Autodesk Inventor part; units mm, degrees
ref_plane "C3_XY" through (128, 0, 0) normal (-1, 0, 0) x (0, 0, -1)
ref_plane "C3_YZ" through (128, 0, 0) normal (0, 0, -1) x (0, -1, 0)
ref_plane "C3_ZX" through (128, 0, 0) normal (0, -1, 0) x (-1, 0, 0)
sketch "Sketch_1" plane through (0, 0, 0) normal (0, 0, 1) x (1, 0, 0)
  line L0 (128, 0) -> (0, 0)
  line L1 (0, 0) -> (0, 3.5)
  line L2 (0, 3.5) -> (0.6062, 4.55)
  line L3 (0.6062, 4.55) -> (127.3938, 4.55)
  line L4 (127.3938, 4.55) -> (128, 3.5)
  line L5 (128, 3.5) -> (128, 0)
  line L6 (128, 0) -> (0, 0)
revolve "Revolution1" add sketch "Sketch_1" angle 360 about axis through (128, 0, 0) along (1, 0, 0)
sketch "Sketch_2" plane through (0, 0, 0) normal (1, 0, 0) x (0, 1, 0)
  line L0 (7, 7) -> (-7, 7)
  line L1 (-7, 7) -> (-7, -7)
  line L2 (-7, -7) -> (7, -7)
  line L3 (7, -7) -> (7, 7)
  line L4 (-2.0207, 3.5) -> (-4.0415, 0)
  line L5 (-4.0415, 0) -> (-2.0207, -3.5)
  line L6 (-2.0207, -3.5) -> (2.0207, -3.5)
  line L7 (2.0207, -3.5) -> (4.0415, 0)
  line L8 (4.0415, 0) -> (2.0207, 3.5)
  line L9 (2.0207, 3.5) -> (-2.0207, 3.5)
extrude "Extrusion1" cut sketch "Sketch_2" along normal blind 128
sketch "Sketch3" plane through (0, 0, 0) normal (-1, 0, 0) x (0, 0, 1)
  point P0 (0, 0)
hole "Hole1" at (0, 0, 0) direction (1, 0, 0) diameter 2.459 depth 8.2901 tip angle 120 countersink diameter 3 countersink angle 90
sketch "Sketch4" plane through (128, 0, 0) normal (1, 0, 0) x (0, 0, -1)
  point P0 (0, 0)
hole "Hole2" at (128, 0, 0) direction (-1, 0, 0) diameter 2.459 depth 8.2901 tip angle 120 countersink diameter 3 countersink angle 90
ref_plane "C3_XY" through (128, 0, 0) normal (-1, 0, 0) x (0, 0, -1)
ref_plane "C3_YZ" through (128, 0, 0) normal (0, 0, -1) x (0, -1, 0)
ref_plane "C3_ZX" through (128, 0, 0) normal (0, -1, 0) x (-1, 0, 0)
properties part number "SLSBF7-128-M3-N3" material "ステンレス鋼 AISI 304"
Geometry check sheet. Reference: the model listing, model coordinates, mm. A direction names the side the tool comes from. Round coordinates to 2 decimals unless told otherwise and drop trailing zeros. Order: outer loops, then holes, each group sorted by start corner. A loop starts at its lowest first (then second) coordinate and runs counter-clockwise, first axis right, second up. Notation, with made-up numbers: (33, 85.25) - (72, 85.25) arc R14 cw to (72, 96.25) - close; hole circle Ø6 at (6.25, -39.5). An arc over 180 degrees is marked (long way). Use a Markdown table: item, result. Add a question column.
1) Thickness scan on line 1 along Y through (x, z) = (4.25, 0); line 2 along Z through (x, y) = (124, 0); line 3 along X through (y, z) = (-3.5, 0.5). Record the ranges inside material, lowest first.
2) Gauge pin test, flat ends, axial feed: P1, Ø1.5, axis at x = 105.5, y = -3, coming from the -Z side; P2, Ø2, axis at y = 0, z = 0, coming from the +X side; P3, Ø1, axis at x = 107, y = -3, coming from the +Z side. Record the tip position at first contact, or that the pin passes through.
3) Section check A-A (x = 80.5). Record the cut outline in (y, z).
4) Set-up check for faces 5 (the flat face through (63.1, 3, -1.8)), 6 (the cylindrical face through (4.336, 0.748, -0.976)): record each of +Z, -Z, +X, -X, +Y, -Y from which the full face is reachable in a straight line by a thin tool's end or side.
5) Mould release check, pull along Y, two halves, no side actions. Record for faces 1 (the flat face through (63.104, -3.045, -1.726)), 2 (the flat face through (0, 0, -2)), 3 (the flat face through (63.104, 3.045, 1.726)), 4 (the cylindrical face through (123.664, 0.748, 0.976)): released by +Y, released by -Y, zero draft, split by the parting line, or undercut.
Established:
| question | item | result |
|---|---|---|
| 1 | line 1 | -4.04 to -1.23, 1.23 to 4.04 |
| 1 | line 2 | -3.5 to -1.23, 1.23 to 3.5 |
| 1 | line 3 | 0.02 to 127.98 |
| 2 | P1 | z = -3.1 |
| 2 | P2 | x = 119.58 |
| 2 | P3 | z = 2.67 |
| 3 | outline | (-4.04, 0) - (-2.02, -3.5) - (2.02, -3.5) - (4.04, 0) - (2.02, 3.5) - (-2.02, 3.5) - close |
| 4 | face 5 | -Z, +X, -X, +Y |
| 4 | face 6 | -X |
| 5 | face 1 | released by -Y |
| 5 | face 2 | zero draft |
| 5 | face 3 | released by +Y |
| 5 | face 4 | undercut |
